from build123d import *

# Parameters (mm, degrees)
SKETCH1_R                       = 19
BOSS_EXTRUDE1_DEPTH             = 35
SKETCH2_R                       = 10
BOSS_EXTRUDE2_DEPTH             = 5
SKETCH3_R                       = 3
BOSS_EXTRUDE3_DEPTH             = 13
CUT_EXTRUDE1_START              = -10
CUT_EXTRUDE1_DEPTH              = 10
TAP_DRILL_FOR_M3X0_5_TAP1_D     = 2.5
TAP_DRILL_FOR_M3X0_5_TAP1_DEPTH = 5
TAP_DRILL_FOR_M3X0_5_TAP1_TIP   = 0.751075774


with BuildPart() as part:
    # Sketch1 → Boss-Extrude1 (new body)
    with BuildSketch(Plane.XY):
        Circle(SKETCH1_R)
    extrude(amount=BOSS_EXTRUDE1_DEPTH)

    # Sketch2 → Boss-Extrude2 (add)
    with BuildSketch(Plane.XY.offset(35)):
        Circle(SKETCH2_R)
    extrude(amount=BOSS_EXTRUDE2_DEPTH)

    # Sketch3 → Boss-Extrude3 (add)
    with BuildSketch(Plane.XY.offset(40)):
        with Locations(Location((0, 0, 0), (0, 0, 180))):
            Circle(SKETCH3_R)
    extrude(amount=BOSS_EXTRUDE3_DEPTH)

    # Sketch4 → Cut-Extrude1 (cut)
    with BuildSketch(Plane.XY.offset(53).offset(CUT_EXTRUDE1_START)):
        with BuildLine():
            Line((-1.658312395, 2.5), (1.658312395, 2.5))
            ThreePointArc((1.658312395, 2.5), (0, 3), (-1.658312395, 2.5))
        make_face()
    extrude(amount=CUT_EXTRUDE1_DEPTH, mode=Mode.SUBTRACT)

    # Tap Drill for M3x0.5 Tap1
    with Locations(Plane.XY.offset(35)):
        with Locations((-15, 0), (0, 14), (7.5, 12.990381057), (12.124355653, -7), (7.5, -12.990381057), (-12.124355653, -7)):
            Hole(TAP_DRILL_FOR_M3X0_5_TAP1_D / 2, depth=TAP_DRILL_FOR_M3X0_5_TAP1_DEPTH)
            with Locations((0, 0, -(TAP_DRILL_FOR_M3X0_5_TAP1_DEPTH + TAP_DRILL_FOR_M3X0_5_TAP1_TIP / 2))):  # 118° drill point
                Cone(0, TAP_DRILL_FOR_M3X0_5_TAP1_D / 2, TAP_DRILL_FOR_M3X0_5_TAP1_TIP, mode=Mode.SUBTRACT)


solid = part.part
Geometry check sheet. Reference: the model listing, model coordinates, mm. A direction names the side the tool comes from. Round coordinates to 2 decimals unless told otherwise and drop trailing zeros. Order: outer loops, then holes, each group sorted by start corner. A loop starts at its lowest first (then second) coordinate and runs counter-clockwise, first axis right, second up. Notation, with made-up numbers: M 78,35.5 L 119,35.5 A26 ccw 119,61.5 Z; hole C 12.25,-13 d10. An arc over 180 degrees is marked long. Answer in a Markdown table with one row per item. Add a question column.
Item 1: Sectioned sample at D-D, the plane z = 36.5. Enter the section's corners in (x, y), plus the area to 3 significant figures.
Item 2: Sectioned sample at A-A, the plane z = 47. Enter the section's corners in (x, y), plus the area to 3 significant figures.
Item 3: Sectioned sample at B-B, the plane x = -5.5. Enter the section's corners in (y, z), plus the area to 3 significant figures.
Item 4: Set-up check for faces 5 (the face through (0, 0, 53)), 6 (the face through (8.75, 13.05, 32.47)), 7 (the face through (0, 2.5, 48)): record each of +Z, -Z, +X, -X, +Y, -Y from which the full face is reachable in a straight line by a thin tool's end or side.
Item 5: Material ranges on L1, parallel to Y at x = 0, z = 32.4; L2, parallel to Y at x = 7, z = 33; L3, parallel to X at y = -7, z = 33.55, recorded low to high. Write a range as [from, to].
Item 6: Sectioned sample at C-C, the plane y = 7. Enter the section's corners in (x, z), plus the area to 3 significant figures.
Item 7: Depth check by flat-ended pin: pin 1 Ø4 at (x, y) = (7.5, -12.99) entering from +Z; pin 2 Ø4 at (x, z) = (6.5, 16) entering from -Y; pin 3 Ø10 at (y, z) = (-14.5, 29) entering from +X; pin 4 Ø10 at (x, y) = (-4.5, 4.5) entering from +Z. Enter the tip coordinate at first touch or a pass-through.
Item 8: Draft check along X on faces 1 (the face through (8.767, -16.856, 17.255)), 2 (the face through (2.1, 2.4, 40)), 3 (the face through (8.75, -12.94, 32.47)), 4 (the face through (0.2, 13.92, 29.38)). Enter one of: released by +X, released by -X, zero draft, split by the parting line, or undercut.
Filled in:
| question | item | result |
|---|---|---|
| 1 | outline | C 0,0 d20 |
| 1 | area | 314 mm² |
| 2 | outline | M -1.66,2.5 A3 ccw long 1.66,2.5 Z |
| 2 | area | 27.1 mm² |
| 3 | outline | M -18.19,0 L 18.19,0 L 18.19,35 L 8.35,35 L 8.35,40 L -8.35,40 L -8.35,35 L -18.19,35 Z |
| 3 | area | 1,360 mm² |
| 4 | face 5 | +Z, +X, -X, +Y, -Y |
| 4 | face 6 | +Z |
| 4 | face 7 | +Z, +X, -X, +Y |
| 5 | L1 | y = [-19, 12.75], [15.25, 19] |
| 5 | L2 | y = [-17.66, -14.14], [-11.84, 11.84], [14.14, 17.66] |
| 5 | L3 | x = [-17.66, -13.37], [-10.87, 10.87], [13.37, 17.66] |
| 6 | outline | M -17.66,0 L 17.66,0 L 17.66,35 L 7.14,35 L 7.14,40 L -7.14,40 L -7.14,35 L -17.66,35 Z |
| 6 | area | 1,310 mm² |
| 7 | pin 1 | stops at z = 35 |
| 7 | pin 2 | stops at y = -18.46 |
| 7 | pin 3 | stops at x = 16.45 |
| 7 | pin 4 | stops at z = 53 |
| 8 | face 1 | split by the parting line |
| 8 | face 2 | zero draft |
| 8 | face 3 | undercut |
| 8 | face 4 | undercut |
